Model file for the job. Use its own axes, mm. A direction names the side the tool comes from. Coordinates: 2 decimals unless noted, no trailing zeros. Write each loop counter-clockwise with the first axis right and the second up, starting at its lowest first coordinate (ties: lowest second). Pieces come first, ordered by that corner, then holes. Notation, with made-up numbers: M 22,58.25 L 44,58.25 A24 cw 44,79.25 Z; hole C 26.25,-34 d5. An arc over 180 degrees is marked long. Use CSV: the item, a comma, the result in double quotes. Start each with the question number.
from build123d import *

# Parameters (mm, degrees)
SKETCH1_R           = 11
BOSS_EXTRUDE1_DEPTH = 7
SKETCH3_R           = 18.5
CUT_EXTRUDE1_DEPTH  = 8
CUT_EXTRUDE3_DEPTH  = 8


with BuildPart() as part:
    # Sketch1 → Boss-Extrude1 (new body)
    with BuildSketch(Plane.XY):
        with BuildLine():
            Line((42.143593539, 104.994845224), (-13.856406461, 8))
            ThreePointArc((-13.856406461, 8), (-13.856406461, -8), (0, -16))
            Line((0, -16), (112, -16))
            ThreePointArc((112, -16), (125.856406461, -8), (125.856406461, 8))
            Line((125.856406461, 8), (69.856406461, 104.994845224))
            ThreePointArc((69.856406461, 104.994845224), (56, 112.994845224), (42.143593539, 104.994845224))
        make_face()
        Circle(SKETCH1_R, mode=Mode.SUBTRACT)
        with Locations((112, 0)):
            Circle(SKETCH1_R, mode=Mode.SUBTRACT)
        with Locations((56, 96.994845224)):
            Circle(SKETCH1_R, mode=Mode.SUBTRACT)
    extrude(amount=BOSS_EXTRUDE1_DEPTH)

    # Sketch3 → Cut-Extrude1 (cut, through all)
    with BuildSketch(Plane.XY.offset(7)):
        with Locations((56, 65.944845224)):
            Circle(SKETCH3_R)
    extrude(amount=-CUT_EXTRUDE1_DEPTH, mode=Mode.SUBTRACT)

    # Sketch6 → Cut-Extrude3 (cut, through all)
    with BuildSketch(Plane.XY):
        with BuildLine():
            Line((23.108803184, 52.025621216), (4.866153476, 20.428425058))
            ThreePointArc((4.866153476, 20.428425058), (18.186533479, 10.5), (20.124611797, -6))
            Line((20.124611797, -6), (51, -6))
            Line((51, -6), (51, 35.922631226))
            Line((51, 35.922631226), (23.108803184, 52.025621216))
        make_face()
        with BuildLine():
            Line((61, 35.922631226), (61, -6))
            Line((61, -6), (91.875388203, -6))
            ThreePointArc((91.875388203, -6), (93.813466521, 10.5), (107.133846524, 20.428425058))
            Line((107.133846524, 20.428425058), (88.891196816, 52.025621216))
            Line((88.891196816, 52.025621216), (61, 35.922631226))
        make_face()
    extrude(amount=CUT_EXTRUDE3_DEPTH, mode=Mode.SUBTRACT)


solid = part.part
1) Wall check: L1, parallel to Y at x = 56, z = 4.5; L2, parallel to Y at x = 107, z = 2; L3, parallel to X at y = 9.5, z = 1.25. Give the ranges that are in metal, low to high. Write a range as [from, to].
2) Band-saw the part on C-C on y = 17. List the corners of the cut face in (x, z).
3) Drop flat-ended pins along their axis: P1, Ø8, axis at x = 70.5, y = 1, coming from the +Z side; P2, Ø1, axis at y = 39.5, z = 6.5, coming from the -X side; P3, Ø3.5, axis at y = 24.5, z = 2.5, coming from the -X side; P4, Ø2, axis at x = 76.5, z = 3.5, coming from the +Y side. Give the stop position or say it passes through.
4) Tool access for faces 1 (the face through (35, -6, 3)), 2 (the face through (98.248, 55.818, 3.451)): list every direction of +Z, -Z, +X, -X, +Y, -Y with a clear straight run to the whole face (end or side of a thin tool).
5) Band-saw the part on D-D on z = 5.25. List the corners of the cut face in (x, y), then the cut area to 3 significant figures.
6) Band-saw the part on B-B on y = 0. List the corners of the cut face in (x, z), then the cut area to 3 significant figures.
7) Band-saw the part on A-A on x = 56. List the corners of the cut face in (y, z).
8) Two-plate mould, pull along Y, no slides. Class faces 3 (the face through (125.74, -8.2, 3.45)), 4 (the face through (75.141, 44.087, 3.451)), 5 (the face through (55, -16, 3)), 6 (the face through (14.115, 36.448, 3.451)): pulls with the +Y half, pulls with the -Y half, needs draft (parallel to the pull), parting line crosses it, or undercut.
Findings below:
1,L1,"y = [-16, 47.44], [84.44, 85.99], [107.99, 112.99]"
1,L2,"y = [-16, -9.8], [9.8, 20.4], [20.66, 40.66]"
1,L3,"x = [-12.99, -5.55], [5.55, 18.73], [51, 61], [93.27, 106.45], [117.55, 124.99]"
2,outline,"M -8.66,0 L 12.33,0 L 12.33,7 L -8.66,7 Z; M 51,0 L 61,0 L 61,7 L 51,7 Z; M 99.67,0 L 120.66,0 L 120.66,7 L 99.67,7 Z"
3,P1,"passes through"
3,P2,"stops at x = 4.04"
3,P3,"stops at x = -5.34"
3,P4,"stops at y = 95.22"
4,face 1,"+Z, -Z"
4,face 2,"+Z, -Z, +X, +Y"
5,outline,"M -13.86,8 A16 ccw 0,-16 L 112,-16 A16 ccw 125.86,8 L 69.86,104.99 A16 ccw 42.14,104.99 Z; hole C 0,0 d22; hole M 4.87,20.43 A21 cw 20.12,-6 L 51,-6 L 51,35.92 L 23.11,52.03 Z; hole C 56,65.94 d37; hole C 56,96.99 d22; hole M 61,-6 L 91.88,-6 A21 cw 107.13,20.43 L 88.89,52.03 L 61,35.92 Z; hole C 112,0 d22"
5,area,"5,750 mm2"
6,outline,"M -16,0 L -11,0 L -11,7 L -16,7 Z; M 11,0 L 21,0 L 21,7 L 11,7 Z; M 51,0 L 61,0 L 61,7 L 51,7 Z; M 91,0 L 101,0 L 101,7 L 91,7 Z; M 123,0 L 128,0 L 128,7 L 123,7 Z"
6,area,"280 mm2"
7,outline,"M -16,0 L 47.44,0 L 47.44,7 L -16,7 Z; M 84.44,0 L 85.99,0 L 85.99,7 L 84.44,7 Z; M 107.99,0 L 112.99,0 L 112.99,7 L 107.99,7 Z"
8,face 3,"parting line crosses it"
8,face 4,"undercut"
8,face 5,"pulls with the -Y half"
8,face 6,"undercut"
